Read the model definition and answer for the solid it produces. Units are mm, in the model's axes. A direction names the side the tool comes from. Coordinates: 2 decimals unless noted, no trailing zeros. Loops run counter-clockwise (first coordinate to the right, second up) from the corner with the lowest first, then second, coordinate; pieces in that order, holes last. Notation, with made-up numbers: M 56,-12 L 86,-12 A19 ccw 86,-1 Z; hole C -3,51 d8. An arc over 180 degrees is marked long. Use one line per item in the form item = value. Start each with the question number.
1. The part is cut by section D-D (z = -8). Give the vertices of the cut face in (x, y), plus the area to 3 significant figures.
2. Find the intervals of material crossed by probe 1 along X at (y, z) = (41, 13); probe 2 along Z at (x, y) = (-17.5, 43); probe 3 along X at (y, z) = (46.5, -12), in increasing order. Write a range as [from, to].
3. The part is cut by section A-A (y = 43). Give the vertices of the cut face in (x, z).
4. A tool of negligible diameter and unlimited length cuts with its end or side. For faces 1 (the flat face through (0, 48, 18)), 2 (the cylindrical face through (-8.643, 45.146, -17.98)), 3 (the cylindrical face through (-12.693, 42.737, 9.564)), from which of +Z, -Z, +X, -X, +Y, -Y can it reach the whole face along a straight path? Write none if from no direction.
5. The part is cut by section C-C (z = 0). Give the vertices of the cut face in (x, y).
6. The part is cut by section B-B (x = 15.5). Give the vertices of the cut face in (y, z).
7. Flat-ended cylindrical pins translate along their axes: pin 1 (9 mm diameter, centred on x = -15, z = -14, fed in from -Y); pin 2 (6 mm diameter, centred on x = 5.5, z = 16.5, fed in from -Y); pin 3 (2 mm diameter, centred on x = -2.5, y = 46, fed in from +Z). Find the tip coordinate at first contact, or state that the pin passes through.
Solid Edge part; units mm, degrees
sketch "Sketch1" plane through (0, 50, 11.75) normal (0, -1, 0) x (1, 0, 0)
  line L0 (-22.5, -33.25) -> (22.5, -33.25)
  line L1 (22.5, 9.75) -> (22.5, -33.25)
  line L2 (22.5, 9.75) -> (-22.5, 9.75)
  line L3 (-22.5, 9.75) -> (-22.5, -33.25)
  dimension "D1" = 22.5
  dimension "D2" = 22.5
extrude "ExtrudedProtrusion_2" add sketch "Sketch1" along normal blind 12
sketch "Sketch2" plane through (0, 0, 0) normal (1, 0, 0) x (0, 1, 0)
  arc A0 (50, -9.5) -> (50, 9.5) centre (50, 0) cw
  line L0 (50, 9.5) -> (50, -9.5)
  dimension "D1" = 50
extrude "Cutout1" cut sketch "Sketch2" along normal through all and the other way through all
sketch "Sketch3" plane through (-22.5, 44, 0) normal (-1, 0, 0) x (0, 0, -1)
  arc A0 (20.6458, 0) -> (21.5, -6) centre (0, -6) cw
  line L0 (27.9876, -6) -> (21.5, -6)
  line L1 (27.9876, 18.1819) -> (27.9876, -6)
  line L2 (-27.4197, 18.1819) -> (27.9876, 18.1819)
  line L3 (-27.4197, -6) -> (-27.4197, 18.1819)
  line L4 (-21.5, -6) -> (-27.4197, -6)
  arc A1 (-21.5, -6) -> (-20.6458, 0) centre (0, -6) cw
  arc A2 (-20.6458, 0) -> (20.6458, 0) centre (0, -34.26) cw
extrude "Cutout2" cut sketch "Sketch3" against normal up to next
sketch "Sketch4" plane through (0, 38, 0) normal (0, -1, 0) x (1, 0, 0)
  circle A0 centre (-15, 14) radius 3
  circle A1 centre (15, 14) radius 3
  circle A2 centre (-15, -14) radius 3
  circle A3 centre (15, -14) radius 3
extrude "Cutout3" cut sketch "Sketch4" against normal through all
sketch "Sketch5" plane through (0, 38, 0) normal (0, -1, 0) x (1, 0, 0)
  circle A0 centre (-15, 14) radius 5
  circle A1 centre (15, 14) radius 5
  circle A2 centre (15, -14) radius 5
  circle A3 centre (-15, -14) radius 5
extrude "Cutout4" cut sketch "Sketch5" against normal blind 7
sketch "Sketch6" plane through (0, 38, 0) normal (0, -1, 0) x (1, 0, 0)
  arc A0 (15, 21.5) -> (7.5, 14) centre (15, 14) ccw
  line L0 (-7.5, 14) -> (7.5, 14)
  arc A1 (-15, 21.5) -> (-7.5, 14) centre (-15, 14) cw
  line L1 (-15, 21.5) -> (15, 21.5)
  arc A2 (15, -21.5) -> (7.5, -14) centre (15, -14) cw
  line L2 (-7.5, -14) -> (7.5, -14)
  arc A3 (-15, -21.5) -> (-7.5, -14) centre (-15, -14) ccw
  line L3 (-15, -21.5) -> (15, -21.5)
extrude "ExtrudedCutout_9" cut sketch "Sketch6" against normal blind 10
properties material "Aluminum, 1060"
Computed values:
q1.outline = M -22.5,39.07 L 22.5,39.07 L 22.5,44.88 L -22.5,44.88 Z
q1.area = 261 mm²
q2.probe_1 = [-22.5, -19.9], [-10.1, 10.1], [19.9, 22.5]
q2.probe_2 = [-18.89, -18.33], [-9.67, -6.42], [6.42, 9.67], [18.33, 18.89]
q2.probe_3 = [-22.5, -17.24], [-12.76, 12.76], [17.24, 22.5]
q3.outline = M -22.5,-18.89 L -16.06,-18.89 A5 cw long -13.94,-18.89 L -9.31,-18.89 A7.5 ccw -7.5,-14 L 7.5,-14 A7.5 ccw 9.31,-18.89 L 13.94,-18.89 A5 cw long 16.06,-18.89 L 22.5,-18.89 L 22.5,-6.42 L -22.5,-6.42 Z; M -22.5,6.42 L 22.5,6.42 L 22.5,18.89 L 16.06,18.89 A5 cw long 13.94,18.89 L 9.31,18.89 A7.5 ccw 7.5,14 L -7.5,14 A7.5 ccw -9.31,18.89 L -13.94,18.89 A5 cw long -16.06,18.89 L -22.5,18.89 Z
q4.face_1 = +Z, -Y
q4.face_2 = -Z, -Y
q4.face_3 = -Y
q5.outline = M -22.5,38.26 L 22.5,38.26 L 22.5,40.5 L -22.5,40.5 Z
q6.outline = M 39.29,-9.03 L 45,-9.03 L 45,-11.04 L 50,-11.04 L 50,-9.5 A9.5 cw 50,9.5 L 50,11.04 L 45,11.04 L 45,9.03 L 39.29,9.03 A40 ccw Z; M 43.05,-18.97 A40 ccw 44,-20.65 A21.5 ccw 50,-21.5 L 50,-16.96 L 45,-16.96 L 45,-18.97 Z; M 43.05,18.97 L 45,18.97 L 45,16.96 L 50,16.96 L 50,21.5 A21.5 ccw 44,20.65 A40 ccw Z
q7.pin_1 = 45
q7.pin_2 = 40.61
q7.pin_3 = 14
